Here's how the part is built. I have some questions about the finished solid (model axes, mm). Give positions to 0.01 mm unless a question says otherwise; leave off trailing zeros. Loops run counter-clockwise (first coordinate to the right, second up) from the corner with the lowest first, then second, coordinate; pieces in that order, holes last.
Q1. Suppose I cut it at B-B (x = 0). Count the separate pieces of the cut face and the enclosed holes in it, and give its area (3 significant figures).
Q2. Suppose I cut it at D-D (y = 0). List the corners of the cut face in (x, z) for me.
Q3. Suppose I cut it at C-C (z = 12.5). List the corners of the cut face in (x, y) for me.
Q4. Thinking about a two-plate mould opening in Y: for faces 1 (the face through (-1.038, 57.004, 8.874)), 2 (the face through (0, 16, 0)), 3 (the face through (0, -69, 9)), 4 (the face through (0, 69, 9)), which applies, pulls with the +Y half, pulls with the -Y half, needs draft (parallel to the pull), parting line crosses it, or undercut?
Q5. I need wall thicknesses on probe 1 along X at (y, z) = (24, 6); probe 2 along X at (y, z) = (60, 11.25). Which ranges of each line are inside material? Lowest first, please.
Q6. I'm going to push a flat-ended pin straight in: P1, Ø4, axis at x = 0, y = 22, coming from the +Z side. Where does the tip first touch, or does it pass through?
Q7. Suppose I cut it at A-A (y = 44). List the corners of the cut face in (x, z) for me, and give its area (3 significant figures).
```python
from build123d import *

# Parameters (mm, degrees)
SKETCH_1_W         = 7
SKETCH_1_H         = 138
EXTRUDE_1_DEPTH    = 18
HOLE_WIZARD_M4_1_D = 4.8
HOLE_WIZARD_M4_2_D = 4.5


with BuildPart() as part:
    # ｽｹｯﾁ1 → ﾎﾞｽ - 押し出し1 (new body)
    with BuildSketch(Plane.XY):
        Rectangle(SKETCH_1_W, SKETCH_1_H)
    extrude(amount=EXTRUDE_1_DEPTH)

    # M4 すきま穴1 (through all)
    with Locations(Plane.XY.offset(18)):
        with Locations((0, 0), (0, 22), (0, -22)):
            Hole(HOLE_WIZARD_M4_1_D / 2)

    # M4 すきま穴2 (through all)
    with Locations(Plane(origin=(0, 44, 18), x_dir=(1, 0, 0), z_dir=(0, 0, 1))):
        with Locations((0, 0), (0, 15)):
            hole_wizard_m4_2 = Hole(HOLE_WIZARD_M4_2_D / 2)

    # ﾐﾗｰ1: M4 すきま穴2 across plane
    add(hole_wizard_m4_2.mirror(Plane.ZX), mode=Mode.SUBTRACT)


solid = part.part
```
Solutions:
1. separate pieces: 8
1. enclosed holes: 0
1. area: 1,900 mm2
2. outline: (-3.5, 0) - (-2.4, 0) - (-2.4, 18) - (-3.5, 18) - close; (2.4, 0) - (3.5, 0) - (3.5, 18) - (2.4, 18) - close
3. outline: (-3.5, -69) - (3.5, -69) - (3.5, 69) - (-3.5, 69) - close; hole circle Ø4.8 at (0, -22); hole circle Ø4.8 at (0, 0); hole circle Ø4.8 at (0, 22); hole circle Ø4.5 at (0, -59); hole circle Ø4.5 at (0, -44); hole circle Ø4.5 at (0, 44); hole circle Ø4.5 at (0, 59)
4. face 1: undercut
4. face 2: needs draft
4. face 3: pulls with the -Y half
4. face 4: pulls with the +Y half
5. probe 1: x = -3.5 to -1.33, 1.33 to 3.5
5. probe 2: x = -3.5 to -2.02, 2.02 to 3.5
6. P1: passes through
7. outline: (-3.5, 0) - (-2.25, 0) - (-2.25, 18) - (-3.5, 18) - close; (2.25, 0) - (3.5, 0) - (3.5, 18) - (2.25, 18) - close
7. area: 45.0 mm2
